Design review of the part built by this model. Coordinates are the model's own, in mm. A direction names the side the tool comes from. Give positions to 0.01 mm unless a question says otherwise; leave off trailing zeros. Loops run counter-clockwise (first coordinate to the right, second up) from the corner with the lowest first, then second, coordinate; pieces in that order, holes last. Notation, with made-up numbers: (-8.5, 28) - (46.5, 28) arc R14 cw to (46.5, 36) - close; hole circle Ø6 at (-18, 3.25). An arc over 180 degrees is marked (long way). Write each question's results on one line, items separated by ' | '.
```python
from build123d import *

# Parameters (mm, degrees)
EXTRUDE1_DEPTH      = 4
EXTRUDE2_DEPTH      = 7
EXTRUDE2_DEPTH_BACK = 16


with BuildPart() as part:
    # Sketch1 → Extrude1 (new, symmetric)
    with BuildSketch(Plane.XY):
        with BuildLine():
            Line((-19, 11.090536506), (-19, 17.748239349))
            ThreePointArc((-19, 17.748239349), (0, 26), (19, 17.748239349))
            Line((19, 17.748239349), (19, 11.090536506))
            ThreePointArc((19, 11.090536506), (0, 22), (-19, 11.090536506))
        make_face()
    extrude(amount=EXTRUDE1_DEPTH, both=True)

    # Sketch2 → Extrude2 (add, two sides: drawn at the far end of the back side and taken through both)
    with BuildSketch(Plane(origin=(0, 0, 4), x_dir=(-1, 0, 0), z_dir=(0, 0, -1)).offset(-EXTRUDE2_DEPTH_BACK)):
        with BuildLine():
            Line((6, 21.685248442), (6, 28.883386228))
            ThreePointArc((6, 28.883386228), (0, 29.5), (-6, 28.883386228))
            Line((-6, 28.883386228), (-6, 21.685248442))
            ThreePointArc((-6, 21.685248442), (0, 22.5), (6, 21.685248442))
        make_face()
    extrude(amount=EXTRUDE2_DEPTH + EXTRUDE2_DEPTH_BACK)


solid = part.part
```
Item 1: Draft analysis for pull direction X (two halves, no side actions). For faces 6 (the face through (-0.1, 29.5, 8.7)), 7 (the face through (0, 22, 0)), 8 (the face through (0.1, 22.4, -4)), state which applies: +X half, -X half, draft (parallel to the pull), parting line (faces both ways), or undercut.
Output values:
face 6: parting line | face 7: undercut | face 8: draft
Item 2: Tool access review of faces 1 (the face through (6, 25, 11)), 2 (the face through (-6, 25, 11)), 3 (the face through (0.1, 22.5, 12.1)), 4 (the face through (0, 26, 20)), 5 (the face through (19, 14, 0)): name each direction out of +Z, -Z, +X, -X, +Y, -Y from which nothing blocks a thin tool from reaching the whole face with its end or side.
Output values:
face 1: +Z, +X, +Y | face 2: +Z, -X, +Y | face 3: +Z, -Y | face 4: +Z, +X, -X, +Y, -Y | face 5: +Z, -Z, +X, +Y, -Y
Item 3: We need section A-A on z = 1. Give the boundary of the cut face in (x, y), then the cut area to 3 significant figures.
Output values:
outline: (-19, 11.09) arc R22 cw to (19, 11.09) - (19, 17.75) arc R26 ccw to (6, 25.3) - (6, 28.88) arc R29.5 ccw to (-6, 28.88) - (-6, 25.3) arc R26 ccw to (-19, 17.75) - close | area: 218 mm²
Item 4: Clearance check with flat-ended pins moving along their axes: P1, Ø3.5, axis at y = 24, z = 6, coming from the +X side; P2, Ø1.5, axis at y = 22.5, z = 11, coming from the -X side; P3, Ø8, axis at x = -2.5, z = 11.5, coming from the -Y side. State where each tip first meets the part, or that it passes through.
Output values:
P1: stops at x = 6 | P2: stops at x = -6 | P3: stops at y = 21.69
Item 5: We need section B-B on y = 21. Give the boundary of the cut face in (x, z).
Output values:
outline: (-15.33, -4) - (-6.56, -4) - (-6.56, 4) - (-15.33, 4) - close; (6.56, -4) - (15.33, -4) - (15.33, 4) - (6.56, 4) - close
Item 6: We need section C-C on x = 4. Give the boundary of the cut face in (y, z), then the cut area to 3 significant figures.
Output values:
outline: (21.63, -4) - (25.69, -4) - (25.69, -3) - (29.23, -3) - (29.23, 20) - (22.14, 20) - (22.14, 4) - (21.63, 4) - close | area: 171 mm²
Item 7: Wall thickness on probe 1 along Z at (x, y) = (-9.5, 23); probe 2 along X at (y, z) = (27.25, 3); probe 3 along Y at (x, z) = (14.5, 1): over which ranges is each line inside the solid? List them lowest first.
Output values:
probe 1: z = -4 to 4 | probe 2: x = -6 to 6 | probe 3: y = 16.55 to 21.58
Item 8: We need section D-D on y = 17. Give the boundary of the cut face in (x, z).
Output values:
outline: (-19, -4) - (-13.96, -4) - (-13.96, 4) - (-19, 4) - close; (13.96, -4) - (19, -4) - (19, 4) - (13.96, 4) - close
